Input: part model. Units: mm. Frame: model coordinates. Face numbers are marked on the shaded views. Give positions to 0.01 mm unless a question says otherwise; leave off trailing zeros. Loops run counter-clockwise (first coordinate to the right, second up) from the corner with the lowest first, then second, coordinate; pieces in that order, holes last.
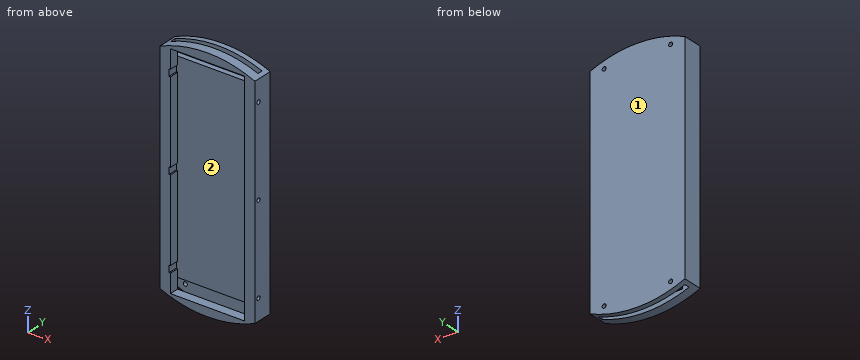
from build123d import *

# Parameters (mm, degrees)
RESSALTO_EXTRUS_O1_DEPTH = 15
CORTE_EXTRUS_O1_DEPTH    = 7
ESBO_O4_W                = 65.5
ESBO_O4_H                = 4
CORTE_EXTRUS_O3_DEPTH    = 14.5
ESBO_O5_W                = 65.5
ESBO_O5_H                = 4
CORTE_EXTRUS_O4_DEPTH    = 14.5
ESBO_O6_R                = 1.5
CORTE_EXTRUS_O5_DEPTH    = 98.99521672
ESBO_O7_R                = 1.5
CORTE_EXTRUS_O6_DEPTH    = 14.5


with BuildPart() as part:
    # Esboço2 → Ressalto-extrusão1 (new body)
    with BuildSketch(Plane(origin=(0, 0, 0), x_dir=(1, 0, 0), z_dir=(0, 1, 0))):
        with BuildLine():
            Line((-35.75, -82.595021036), (-35.75, 82.595021036))
            ThreePointArc((-35.75, 82.595021036), (0, 90), (35.75, 82.595021036))
            Line((35.75, 82.595021036), (35.75, -82.595021036))
            ThreePointArc((35.75, -82.595021036), (0, -90), (-35.75, -82.595021036))
        make_face()
    extrude(amount=RESSALTO_EXTRUS_O1_DEPTH)

    # Esboço3 → Corte-extrusão1 (cut)
    with BuildSketch(Plane(origin=(0, 0, 0), x_dir=(-1, 0, 0), z_dir=(0, -1, 0))):
        Polygon((27.75, 69.5), (27.75, 83.5), (-27.75, 83.5), (-27.75, -83.5), (27.75, -83.5), (27.75, -69.5), (28.75, -69.5), (28.75, -64.4), (27.75, -64.4), (27.75, -2.55), (28.75, -2.55), (28.75, 2.55), (27.75, 2.55), (27.75, 64.4), (28.75, 64.4), (28.75, 69.5), align=None)
    extrude(amount=-CORTE_EXTRUS_O1_DEPTH, mode=Mode.SUBTRACT)

    # Esboço4 → Corte-extrusão3 (cut)
    with BuildSketch(Plane(origin=(0, 0, -90), x_dir=(-1, 0, 0), z_dir=(0, 0, -1))):
        with Locations((0, 9)):
            Rectangle(ESBO_O4_W, ESBO_O4_H)
    extrude(amount=-CORTE_EXTRUS_O3_DEPTH, mode=Mode.SUBTRACT)

    # Esboço5 → Corte-extrusão4 (cut)
    with BuildSketch(Plane.XY.offset(90)):
        with Locations((0, 9)):
            Rectangle(ESBO_O5_W, ESBO_O5_H)
    extrude(amount=-CORTE_EXTRUS_O4_DEPTH, mode=Mode.SUBTRACT)

    # Esboço6 → Corte-extrusão5 (cut, through all)
    with BuildSketch(Plane(origin=(0, 15, 0), x_dir=(1, 0, 0), z_dir=(0, 1, 0))):
        with Locations(Location((-25.01, 80.825021036, 0), (0, 0, 270))):
            Circle(ESBO_O6_R)
        with Locations(Location((25.01, 80.825021036, 0), (0, 0, 270))):
            Circle(ESBO_O6_R)
        with Locations(Location((-25.01, -80.825021036, 0), (0, 0, 270))):
            Circle(ESBO_O6_R)
        with Locations(Location((25.01, -80.825021036, 0), (0, 0, 270))):
            Circle(ESBO_O6_R)
    extrude(amount=-CORTE_EXTRUS_O5_DEPTH, mode=Mode.SUBTRACT)

    # Esboço7 → Corte-extrusão6 (cut)
    with BuildSketch(Plane(origin=(35.75, 0, 0), x_dir=(0, 0, -1), z_dir=(1, 0, 0))):
        with Locations((-66.954978964, 3.5)):
            Circle(ESBO_O7_R)
        with Locations((-0.004978964, 3.5)):
            Circle(ESBO_O7_R)
        with Locations((66.845021036, 3.5)):
            Circle(ESBO_O7_R)
    extrude(amount=-CORTE_EXTRUS_O6_DEPTH, mode=Mode.SUBTRACT)


solid = part.part
(1) Mould query, pull axis X, two halves, no side actions, for the marked faces 1 and 2. Classes: +X half, -X half, draft (parallel to the pull), parting line (faces both ways), or undercut.
Values follow:
face 1: draft
face 2: undercut
(2) Ray query, probe 1 along X at (y, z) = (2, -62); probe 2 along Y at (x, z) = (-10, -9); probe 3 along Y at (x, z) = (-6.5, 78). Return the intervals inside material, ascending.
Values follow:
probe 1: x = -35.75 to -27.75, 27.75 to 35.75
probe 2: y = 7 to 15
probe 3: y = 11 to 15
(3) Cut plane A-A (x = 16). Return the cut outline in (y, z).
Values follow:
outline: (0, -88.57) - (7, -88.57) - (7, -83.5) - (0, -83.5) - close; (0, 83.5) - (7, 83.5) - (7, 88.57) - (0, 88.57) - close; (7, -75.5) - (11, -75.5) - (11, -88.57) - (15, -88.57) - (15, 88.57) - (11, 88.57) - (11, 75.5) - (7, 75.5) - close
(4) Cut plane B-B (z = 15). Return the cut outline in (x, y).
Values follow:
outline: (-35.75, 0) - (-27.75, 0) - (-27.75, 7) - (27.75, 7) - (27.75, 0) - (35.75, 0) - (35.75, 15) - (-35.75, 15) - close
(5) Pin query (flat end, axial travel): pin 1 Ø0.5 at (x, y) = (-28.5, 3) entering from +Z; pin 2 Ø1.1 at (x, y) = (-28, 4.5) entering from -Z; pin 3 Ø12 at (x, z) = (-5.5, 34) entering from -Y; pin 4 Ø1.8 at (x, z) = (-25.01, 80.83) entering from -Y. Return the tip coordinate at first contact, or that it passes through.
Values follow:
pin 1: stops at z = 85.45
pin 2: stops at z = -85.71
pin 3: stops at y = 7
pin 4: passes through
